from build123d import *

# Parameters (mm, degrees)
SKETCH12_W                                      = 20
SKETCH12_H                                      = 30
SKETCH12_R                                      = 5.125
SKETCH12_R_2                                    = 1.7
BOSS_EXTRUDE3_DEPTH                             = 3.18
CSK_FOR_M2_FLAT_HEAD_MACHINE_SCREW2_D           = 2.4
CSK_FOR_M2_FLAT_HEAD_MACHINE_SCREW2_CSINK_D     = 4.4
CSK_FOR_M2_FLAT_HEAD_MACHINE_SCREW2_CSINK_ANGLE = 90
CHAMFER1_SIZE                                   = 1.8
FILLET3_R                                       = 0.5
FILLET4_R                                       = 2


with BuildPart() as part:
    # Sketch12 → Boss-Extrude3 (new body)
    with BuildSketch(Plane.XY):
        with Locations((-10, -15)):
            Rectangle(SKETCH12_W, SKETCH12_H)
        with Locations(Location((-9, -22, 0), (0, 0, 180))):
            Circle(SKETCH12_R, mode=Mode.SUBTRACT)
        with Locations(Location((-5, -6.5, 0), (0, 0, 180))):
            Circle(SKETCH12_R_2, mode=Mode.SUBTRACT)
        with Locations(Location((-15, -8.5, 0), (0, 0, 180))):
            Circle(SKETCH12_R_2, mode=Mode.SUBTRACT)
    extrude(amount=BOSS_EXTRUDE3_DEPTH)

    # CSK for M2 Flat Head Machine Screw2 (through all)
    with Locations(Plane.XY.offset(3.18)):
        with Locations((-9, -15.5), (-14.629165125, -25.25), (-3.370834875, -25.25)):
            CounterSinkHole(CSK_FOR_M2_FLAT_HEAD_MACHINE_SCREW2_D / 2, CSK_FOR_M2_FLAT_HEAD_MACHINE_SCREW2_CSINK_D / 2, counter_sink_angle=CSK_FOR_M2_FLAT_HEAD_MACHINE_SCREW2_CSINK_ANGLE)

    # Chamfer1
    chamfer1_edges = [part.edges().sort_by_distance(p)[0] for p in [
        (-20, 0, 1.59),
        (0, 0, 1.59),
    ]]
    chamfer(chamfer1_edges, length=CHAMFER1_SIZE)

    # Fillet3
    fillet3_edges = [part.edges().sort_by_distance(p)[0] for p in [
        (-20, -1.8, 1.59),
        (0, -1.8, 1.59),
    ]]
    fillet(fillet3_edges, radius=FILLET3_R)

    # Fillet4
    fillet4_edges = [part.edges().sort_by_distance(p)[0] for p in [
        (0, -30, 1.59),
        (-20, -30, 1.59),
    ]]
    fillet(fillet4_edges, radius=FILLET4_R)


solid = part.part
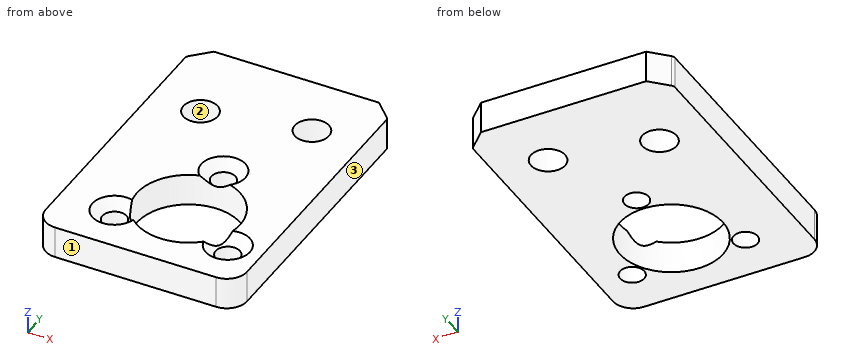
Check sheet for the modelled part. Datum: model origin and axes. Units: mm. Face numbers are marked on the shaded views. Round coordinates to 2 decimals unless told otherwise and drop trailing zeros. Write each loop counter-clockwise with the first axis right and the second up, starting at its lowest first coordinate (ties: lowest second). Pieces come first, ordered by that corner, then holes. Notation, with made-up numbers: (85.5, 11) -> (109.5, 11) arc R27 ccw to (109.5, 27) -> close; hole circle Ø4 at (5.5, 45). An arc over 180 degrees is marked (long way). Answer as CSV lines item,"result". Start each with the question number.
1) Section check C-C on x = -9. Enter the section's corners in (y, z) (3 decimals).
2) Release check for a two-part mould opening along X. For the marked faces 1, 2 and 3 record: pulls with the +X half, pulls with the -X half, needs draft (parallel to the pull), parting line crosses it, or undercut.
3) Material ranges on line 1 (Y direction, x = -9, z = 0.9) (3 decimals); line 2 (Y direction, x = -15, z = 1.9); line 3 (X direction, y = -22, z = 2.15) (3 decimals), recorded low to high. Write a range as from..to.
4) Go/stop test with a flat-tipped pin: P1, Ø1.4, axis at x = -9, y = -15.5, coming from the +Z side. Record where the tip stops, or that it passes through.
5) Section check D-D on y = -25.25. Enter the section's corners in (x, z).
6) Section check B-B on y = -6.5. Enter the section's corners in (x, z), and give its area (3 significant figures).
7) Section check A-A on z = 1.85. Enter the section's corners in (x, y) (3 decimals), and give its area (3 significant figures).
Found:
1,outline,"(-30, 0) -> (-27.125, 0) -> (-27.125, 3.18) -> (-30, 3.18) -> close; (-16.875, 0) -> (-16.7, 0) -> (-16.7, 2.18) -> (-16.875, 2.355) -> close; (-14.3, 0) -> (0, 0) -> (0, 3.18) -> (-13.3, 3.18) -> (-14.3, 2.18) -> close"
2,face 1,"needs draft"
2,face 2,"undercut"
2,face 3,"pulls with the +X half"
3,line 1,"y = -30..-27.125, -16.875..-16.7, -14.3..0"
3,line 2,"y = -30..-26.39, -24.11..-10.2, -6.8..0"
3,line 3,"x = -20..-14.125, -3.875..0"
4,P1,"passes through"
5,outline,"(-20, 0) -> (-15.83, 0) -> (-15.83, 2.18) -> (-16.83, 3.18) -> (-20, 3.18) -> close; (-13.43, 0) -> (-12.96, 0) -> (-12.96, 2.65) -> (-13.43, 2.18) -> close; (-5.04, 0) -> (-4.57, 0) -> (-4.57, 2.18) -> (-5.04, 2.65) -> close; (-2.17, 0) -> (0, 0) -> (0, 3.18) -> (-1.17, 3.18) -> (-2.17, 2.18) -> close"
6,outline,"(-20, 0) -> (-6.7, 0) -> (-6.7, 3.18) -> (-20, 3.18) -> close; (-3.3, 0) -> (0, 0) -> (0, 3.18) -> (-3.3, 3.18) -> close"
6,area,"52.8 mm^2"
7,outline,"(-20, -28) arc R2 ccw to (-18, -30) -> (-2, -30) arc R2 ccw to (0, -28) -> (0, -2.007) arc R0.5 ccw to (-0.146, -1.654) -> (-1.8, 0) -> (-18.2, 0) -> (-19.854, -1.654) arc R0.5 ccw to (-20, -2.007) -> close; hole circle Ø3.4 at (-15, -8.5); hole circle Ø2.4 at (-14.629, -25.25); hole circle Ø10.25 at (-9, -22); hole circle Ø2.4 at (-9, -15.5); hole circle Ø3.4 at (-5, -6.5); hole circle Ø2.4 at (-3.371, -25.25)"
7,area,"481 mm^2"
